from build123d import *

# Parameters (mm, degrees)
SKETCH1_R           = 17
BOSS_EXTRUDE1_DEPTH = 3.5
SKETCH3_R           = 17
BOSS_EXTRUDE2_DEPTH = 3.5
SKETCH4_R           = 6
BOSS_EXTRUDE3_DEPTH = 10


with BuildPart() as part:
    # Sketch1 → Boss-Extrude1 (new, symmetric)
    with BuildSketch(Plane.XY):
        with BuildLine():
            Line((25, 0), (25, -25))
            Line((25, -25), (-47, -25))
            Line((-47, -25), (-47, -9))
            Line((-47, -9), (-43, -9))
            Line((-43, -9), (-43, -5))
            Line((-43, -5), (-16.69831871, 18.605540902))
            ThreePointArc((-16.69831871, 18.605540902), (10.186805983, 22.830439853), (25, 0))
        make_face()
        Circle(SKETCH1_R, mode=Mode.SUBTRACT)
    extrude(amount=BOSS_EXTRUDE1_DEPTH, both=True)

    # Sketch3 → Boss-Extrude2 (add)
    with BuildSketch(Plane.XY.offset(3.5)):
        with BuildLine():
            Line((25, -25), (25, 0))
            ThreePointArc((25, 0), (-11.180339887, 22.360679775), (-15, -20))
            Line((-15, -20), (-15, -25))
            Line((-15, -25), (25, -25))
        make_face()
        Circle(SKETCH3_R, mode=Mode.SUBTRACT)
    boss_extrude2 = extrude(amount=BOSS_EXTRUDE2_DEPTH)

    # Mirror1: Boss-Extrude2 across plane
    add(boss_extrude2.mirror(Plane.XY))

    # Sketch4 → Boss-Extrude3 (add)
    with BuildSketch(Plane.ZY.offset(43)):
        with BuildLine():
            Line((3.5, -5), (16.5, -5))
            ThreePointArc((16.5, -5), (26.5, -15), (16.5, -25))
            Line((16.5, -25), (3.5, -25))
            Line((3.5, -25), (3.5, -5))
        make_face()
        with Locations((16.5, -15)):
            Circle(SKETCH4_R, mode=Mode.SUBTRACT)
    extrude(amount=-BOSS_EXTRUDE3_DEPTH)


solid = part.part
Input: part model. Units: mm. Frame: model coordinates. A direction names the side the tool comes from. Coordinates: 2 decimals unless noted, no trailing zeros. Order: outer loops, then holes, each group sorted by start corner. A loop starts at its lowest first (then second) coordinate and runs counter-clockwise, first axis right, second up. Notation, with made-up numbers: M -14,-6.5 L -8,-6.5 A21 ccw -8,9.5 Z; hole C 20.5,81.5 d10. An arc over 180 degrees is marked long. Write item = value, one per line. Start each with the question number.
(1) Section D-D on z = 18. Output: boundary loops of the cut face in (x, y), and give its area (3 significant figures).
(2) First-contact query: P1, Ø1.8, axis at y = -21.5, z = -5, coming from the -X side; P2, Ø5, axis at x = -20, z = 4.5, coming from the +Y side; P3, Ø4, axis at y = -16.5, z = 14.5, coming from the +X side; P4, Ø10, axis at y = -2.5, z = 11.5, coming from the -X side. Flat tips, straight axial feed; report the tip coordinate or a pass-through.
(3) Section A-A on z = -1. Output: boundary loops of the cut face in (x, y).
(4) Line query: line 1 along Y through (x, z) = (0, 0); line 2 along Y through (x, z) = (-38, 16.5); line 3 along Y through (x, z) = (-41.5, 6.5). Output: solid intervals per line, ascending. Write a range as [from, to].
(5) Section C-C on y = -15. Output: boundary loops of the cut face in (x, z), and give its area (3 significant figures).
(6) Reachability of faces 1 (the flat face through (-5.9, -16.3, 7)), 2 (the flat face through (-15, -22, -5)), 3 (the flat face through (-45, -9, 0)), 4 (the flat face through (-15, -22, 5)), 5 (the flat face through (-33, -15, 10)) from +Z, -Z, +X, -X, +Y, -Y: full face, straight path, thin tool, end or side. Return the list, or none.
(7) Pull-direction query (Y, two-part tool) for faces 6 (the flat face through (-38, -5, 10)), 7 (the flat face through (-45, -17, 3.5)), 8 (the cylindrical face through (9.139, 14.334, 0.098)); classes: released by +Y, released by -Y, zero draft, split by the parting line, or undercut.
(8) Section B-B on x = 0. Output: boundary loops of the cut face in (y, z), and give its area (3 significant figures).
Result set:
q1.outline = M -43,-24.89 L -33,-24.89 L -33,-20.81 L -43,-20.81 Z; M -43,-9.19 L -33,-9.19 L -33,-5.11 L -43,-5.11 Z
q1.area = 81.5 mm²
q2.P1 = -15
q2.P2 = 17.85
q2.P3 = through
q2.P4 = -43
q3.outline = M -47,-25 L 25,-25 L 25,0 A25 ccw -16.7,18.61 L -43,-5 L -43,-9 L -47,-9 Z; hole C 0,0 d34
q4.line_1 = [-25, -17], [17, 25]
q4.line_2 = [-25, -21], [-9, -5]
q4.line_3 = [-25, -5]
q5.outline = M -47,-3.5 L -20,-3.5 L -20,-7 L -8,-7 L -8,7 L -20,7 L -20,3.5 L -33,3.5 L -33,10.5 L -43,10.5 L -43,3.5 L -47,3.5 Z; M -43,22.5 L -33,22.5 L -33,26.5 L -43,26.5 Z; M 8,-7 L 25,-7 L 25,7 L 8,7 Z
q5.area = 705 mm²
q6.face_1 = +Z, +X, +Y, -Y
q6.face_2 = -Z, -X, -Y
q6.face_3 = +Z, -Z, -X, +Y
q6.face_4 = +Z, -Y
q6.face_5 = +Z, +Y, -Y
q7.face_6 = released by +Y
q7.face_7 = zero draft
q7.face_8 = undercut
q8.outline = M -25,-7 L -17,-7 L -17,7 L -25,7 Z; M 17,-7 L 25,-7 L 25,7 L 17,7 Z
q8.area = 224 mm²
